Could you check a few things on this model? Use its own coordinates, in mm. Face numbers are marked on the shaded views. Coordinates: 2 decimals unless noted, no trailing zeros. Loops run counter-clockwise (first coordinate to the right, second up) from the corner with the lowest first, then second, coordinate; pieces in that order, holes last.
1) Imagine slicing it at D-D on x = 4.75. Please give me the cut outline in (y, z), plus the area to 3 significant figures.
2) Imagine slicing it at B-B on y = 2.5. Please give me the cut outline in (x, z), plus the area to 3 significant figures.
3) Imagine slicing it at C-C on z = 44. Please give me the cut outline in (x, y).
4) Thinking about a two-plate mould opening in Z: for the marked faces 1, 2 and 3, which applies, released by +Z, released by -Z, zero draft, split by the parting line, or undercut?
5) If I drill on line 1 along Z through (x, y) = (-0.5, -0.5); line 2 along Z through (x, y) = (1, -1.25); line 3 along X through (y, z) = (-2.75, 16.5), over which ranges is the centre line in solid material (lowest first)?
6) Will this pin go through, and if not, where does the flat tip stop? P1, Ø5, axis at y = -6, z = 5.5, coming from the +X side.
7) Imagine slicing it at A-A on x = -0.5. Please give me the cut outline in (y, z).
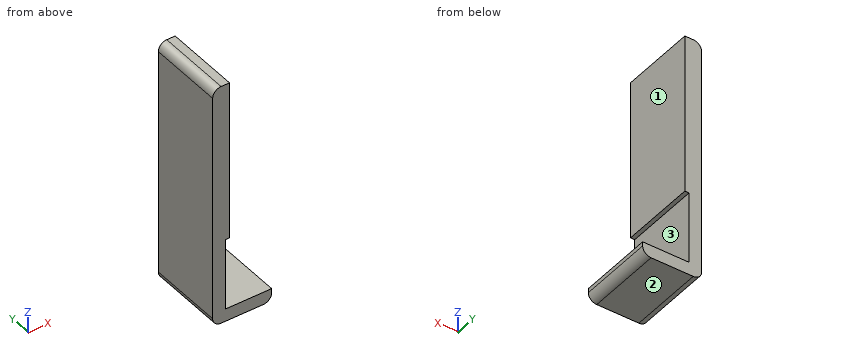
```python
from build123d import *

# Parameters (mm, degrees)
F1_DEPTH = 9
F2_R     = 2
F3_W     = 18
F3_H     = 17
F4_DEPTH = 1


with BuildPart() as f1:
    # F0 (on Front) → F1 (new body, symmetric)
    with BuildSketch(Plane.XZ):
        Polygon((10, 0), (0, 0), (0, 55), (-4, 55), (-4, -3), (10, -3), align=None)
    extrude(amount=F1_DEPTH, both=True)

    # F2
    f2_edges = [f1.edges().sort_by_distance(p)[0] for p in [
        (-4, 0, 55),
        (-4, 0, -3),
        (10, 0, -3),
    ]]
    fillet(f2_edges, radius=F2_R)

    # F3 (on face) → F4 (cut)
    with BuildSketch(Plane.YZ):
        with Locations((0, 8.5)):
            Rectangle(F3_W, F3_H)
    extrude(amount=-F4_DEPTH, mode=Mode.SUBTRACT)


solid = f1.part
```
Filled in:
1. outline: (-9, -3) - (9, -3) - (9, 0) - (-9, 0) - close
1. area: 54.0 mm2
2. outline: (-4, -1) arc R2 ccw to (-2, -3) - (8, -3) arc R2 ccw to (10, -1) - (10, 0) - (-1, 0) - (-1, 17) - (0, 17) - (0, 55) - (-2, 55) arc R2 ccw to (-4, 53) - close
2. area: 242 mm2
3. outline: (-4, -9) - (0, -9) - (0, 9) - (-4, 9) - close
4. face 1: zero draft
4. face 2: released by -Z
4. face 3: undercut
5. line 1: z = -3 to 0, 17 to 55
5. line 2: z = -3 to 0
5. line 3: x = -4 to -1
6. P1: stops at x = -1
7. outline: (-9, -3) - (9, -3) - (9, 0) - (-9, 0) - close; (-9, 17) - (9, 17) - (9, 55) - (-9, 55) - close
